from build123d import *

# Parameters (mm, degrees)
SKETCH010_W     = 44
SKETCH010_H     = 23.4
PAD006_DEPTH    = 2.75
THICKNESS002_T  = 1
SKETCH011_W     = 23.4
SKETCH011_H     = 1
POCKET002_DEPTH = 1
SKETCH012_R     = 2.3
POCKET003_DEPTH = 1
PAD007_DEPTH    = 2.75
SKETCH014_W     = 2
SKETCH014_H     = 23.4
PAD008_DEPTH    = 2


with BuildPart() as part:
    # Sketch010 → Pad006 (new body)
    with BuildSketch(Plane.XY):
        Rectangle(SKETCH010_W, SKETCH010_H)
    extrude(amount=PAD006_DEPTH)

    # Thickness002
    thickness002_openings = [part.faces().sort_by_distance(p)[0] for p in [
        (0, 0, 2.75),
    ]]
    offset(amount=THICKNESS002_T, openings=thickness002_openings)

    # Sketch011 (on Face7 of Thickness002) → Pocket002 (cut)
    with BuildSketch(Plane.YZ.offset(23)):
        with Locations((0, 2.25)):
            Rectangle(SKETCH011_W, SKETCH011_H)
    extrude(amount=-POCKET002_DEPTH, mode=Mode.SUBTRACT)

    # Sketch012 (on Face15 of Pocket002) → Pocket003 (cut)
    with BuildSketch(Plane(origin=(-23, 0, 0), x_dir=(0, -1, 0), z_dir=(-1, 0, 0))):
        with Locations((0, 2.75)):
            Circle(SKETCH012_R)
    extrude(amount=-POCKET003_DEPTH, mode=Mode.SUBTRACT)

    # Sketch013 (on Face2 of Pocket003) → Pad007 (join)
    with BuildSketch(Plane.XY):
        with BuildLine():
            ThreePointArc((10.8, 11.7), (12, 10.5), (13.2, 11.7))
            Line((10.8, 11.7), (13.2, 11.7))
        make_face()
        with BuildLine():
            ThreePointArc((13.2, -11.7), (12, -10.5), (10.8, -11.7))
            Line((10.8, -11.7), (13.2, -11.7))
        make_face()
    extrude(amount=PAD007_DEPTH)

    # Sketch014 (on Face2 of Pad007) → Pad008 (join)
    with BuildSketch(Plane.XY):
        with Locations((-5.2, 0)):
            Rectangle(SKETCH014_W, SKETCH014_H)
    extrude(amount=PAD008_DEPTH)


solid = part.part
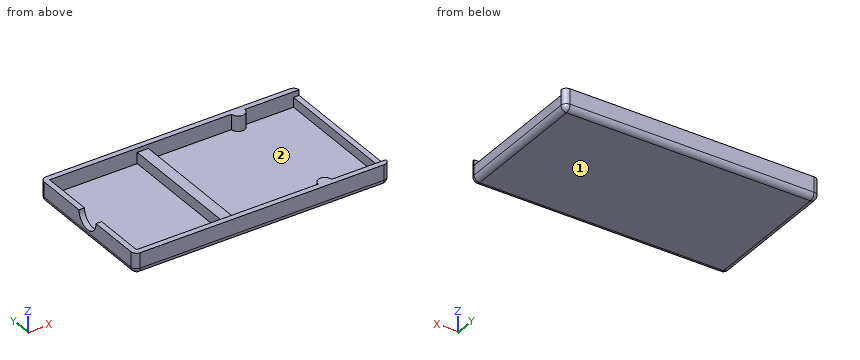
Here's how the part is built. I have some questions about the finished solid (model axes, mm). Face numbers are marked on the shaded views. Round coordinates to 2 decimals unless told otherwise and drop trailing zeros. Write each loop counter-clockwise with the first axis right and the second up, starting at its lowest first coordinate (ties: lowest second). Pieces come first, ordered by that corner, then holes.
1. Will these pins go through, and if not, where does the flat tip stop? pin 1 Ø0.8 at (x, y) = (22.5, -4) entering from +Z; pin 2 Ø4.5 at (x, y) = (-10.5, 0.5) entering from +Z; pin 3 Ø1.6 at (x, y) = (-5, 2.5) entering from +Z.
2. Suppose I cut it at C-C (z = 1.3). List the corners of the cut face in (x, y) for me, and give its area (3 significant figures).
3. Suppose I cut it at A-A (x = 12). List the corners of the cut face in (y, z) for me.
4. Suppose I cut it at D-D (x = 0). List the corners of the cut face in (y, z) for me, and give its area (3 significant figures).
5. If we mould it in two halves opening along Y, with no side actions, what happens to the marked faces 1 and 2? For each: released by +Y, released by -Y, zero draft, split by the parting line, or undercut.
6. I need wall thicknesses on L1, parallel to X at y = -3.25, z = 1.4; L2, parallel to Y at x = -12, z = 0.75; L3, parallel to X at y = 1.5, z = 1.45. Which ranges of each line are inside material? Lowest first, please.
7. Suppose I cut it at B-B (y = 7). List the corners of the cut face in (x, z) for me.
Answer sheet:
1. pin 1: stops at z = 1.75
1. pin 2: stops at z = 0
1. pin 3: stops at z = 2
2. outline: (-23, -11.7) arc R1 ccw to (-22, -12.7) - (22, -12.7) arc R1 ccw to (23, -11.7) - (23, 11.7) arc R1 ccw to (22, 12.7) - (-22, 12.7) arc R1 ccw to (-23, 11.7) - (-23, 1.79) - (-22, 1.79) - (-22, 11.7) - (-6.2, 11.7) - (-6.2, -11.7) - (-22, -11.7) - (-22, -1.79) - (-23, -1.79) - close; hole (-4.2, -11.7) - (10.8, -11.7) arc R1.2 cw to (13.2, -11.7) - (22, -11.7) - (22, 11.7) - (13.2, 11.7) arc R1.2 cw to (10.8, 11.7) - (-4.2, 11.7) - close
2. area: 186 mm2
3. outline: (-12.7, 0) arc R1 ccw to (-11.7, -1) - (11.7, -1) arc R1 ccw to (12.7, 0) - (12.7, 2.75) - (10.5, 2.75) - (10.5, 0) - (-10.5, 0) - (-10.5, 2.75) - (-12.7, 2.75) - close
4. outline: (-12.7, 0) arc R1 ccw to (-11.7, -1) - (11.7, -1) arc R1 ccw to (12.7, 0) - (12.7, 2.75) - (11.7, 2.75) - (11.7, 0) - (-11.7, 0) - (-11.7, 2.75) - (-12.7, 2.75) - close
4. area: 30.5 mm2
5. face 1: zero draft
5. face 2: undercut
6. L1: x = -23 to -22, -6.2 to -4.2, 22 to 23
6. L2: y = -12.7 to -11.7, 11.7 to 12.7
6. L3: x = -6.2 to -4.2, 22 to 23
7. outline: (-23, 0) arc R1 ccw to (-22, -1) - (22, -1) arc R1 ccw to (23, 0) - (23, 1.75) - (22, 1.75) - (22, 0) - (-4.2, 0) - (-4.2, 2) - (-6.2, 2) - (-6.2, 0) - (-22, 0) - (-22, 2.75) - (-23, 2.75) - close
